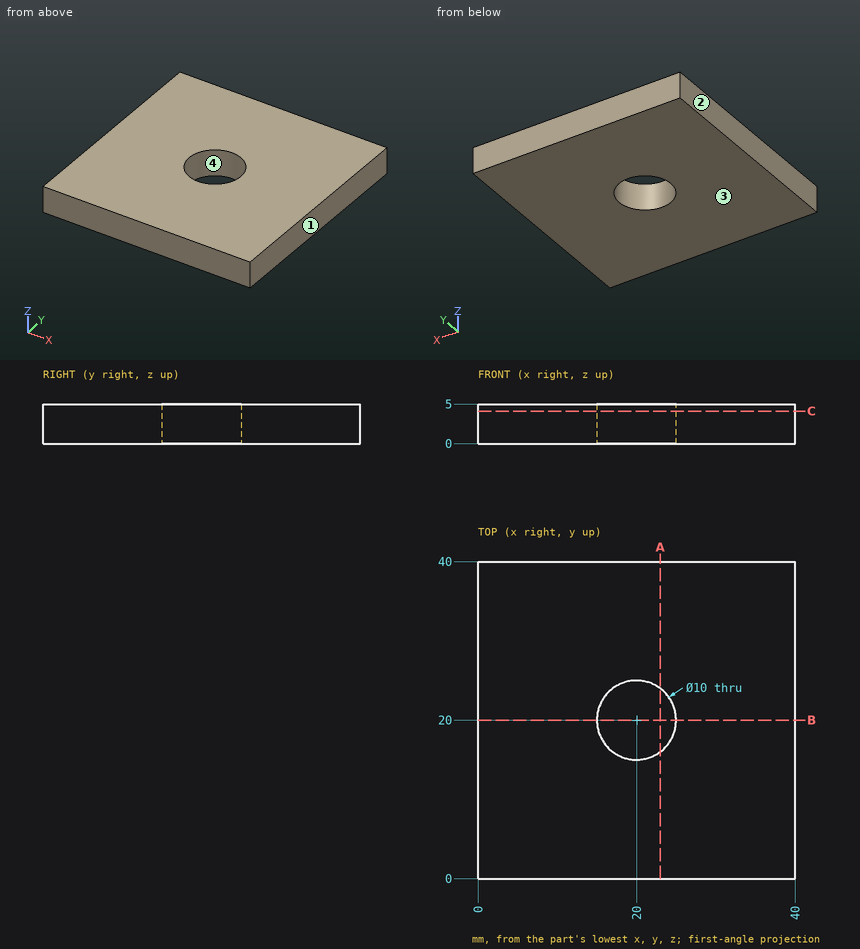
The figure shows three views and two pictorial views of one solid part (mm, origin at its lowest corner). Answer the questions. Coordinates: 2 decimals unless noted, no trailing zeros. Write each loop counter-clockwise with the first axis right and the second up, starting at its lowest first coordinate (ties: lowest second). Pieces come first, ordered by that corner, then holes. Notation, with made-up numbers: M 19,27 L 28,27 A30 ccw 28,63 Z; hole C 24,31.5 d8. An arc over 180 degrees is marked long. Answer as CSV lines item,"result". Start each with the question number.
Item 1: Consider L1, parallel to Y at x = 20, z = 1.75; L2, parallel to Y at x = 24, z = 1.1; L3, parallel to X at y = 22, z = 2. Determine where each line is inside the solid, lowest interval first.
Item 2: A flat-ended cylindrical pin translates along its axis: P1, Ø4, axis at x = 5.5, y = 23.5, coming from the -Z side. Find the tip coordinate at first contact, or state that the pin passes through.
Item 3: Section C-C on z = 4.1 is taken. Write down the section's boundary in (x, y).
Item 4: Section A-A on x = 23 is taken. Write down the section's boundary in (y, z).
Item 5: Section B-B on y = 20 is taken. Write down the section's boundary in (x, z).
Item 6: Determine the mould class of the marked faces 1, 2, 3 and 4 for opening direction X: released by +X, released by -X, zero draft, split by the parting line, or undercut.
Checks:
1,L1,"y = 0 to 15, 25 to 40"
1,L2,"y = 0 to 17, 23 to 40"
1,L3,"x = 0 to 15.42, 24.58 to 40"
2,P1,"stops at z = 0"
3,outline,"M 0,0 L 40,0 L 40,40 L 0,40 Z; hole C 20,20 d10"
4,outline,"M 0,0 L 16,0 L 16,5 L 0,5 Z; M 24,0 L 40,0 L 40,5 L 24,5 Z"
5,outline,"M 0,0 L 15,0 L 15,5 L 0,5 Z; M 25,0 L 40,0 L 40,5 L 25,5 Z"
6,face 1,"released by +X"
6,face 2,"released by -X"
6,face 3,"zero draft"
6,face 4,"undercut"
